Read the model definition and answer for the solid it produces. Units are mm, in the model's axes. Coordinates: 2 decimals unless noted, no trailing zeros. Loops run counter-clockwise (first coordinate to the right, second up) from the corner with the lowest first, then second, coordinate; pieces in that order, holes last.
Q1. Section D-D (x = 6.75) is taken. Give the vertices of the cut face in (y, z).
Q2. Straight lines are drawn through the part: line 1 (Z direction, x = 0.5, y = 25.5); line 2 (Y direction, x = 7.5, z = -23); line 3 (Z direction, x = 4.25, y = 12). For each, find the intervals that lie inside material, in ascending order.
Q3. Section A-A (y = 0) is taken. Give the vertices of the cut face in (x, z).
Q4. Section C-C (y = 22.5) is taken. Give the vertices of the cut face in (x, z).
Q5. The mould has two halves that part along Y. Classify faces 1 (the face through (4.056, 25.203, -22.098)), 2 (the face through (3.94, -39.05, 8.67)), 3 (the face through (0, -26.1, 9.4)), 4 (the face through (4.056, -26.846, 5.961)): pulls with the +Y half, pulls with the -Y half, needs draft (parallel to the pull), parting line crosses it, or undercut.
Q6. A flat-ended cylindrical pin translates along its axis: P1, Ø4, axis at x = 2.5, z = 12, coming from the -Y side. Find the tip coordinate at first contact, or state that the pin passes through.
from build123d import *

# Parameters (mm, degrees)
SKETCH1_R           = 40
BOSS_EXTRUDE1_DEPTH = 8
SKETCH3_R           = 4
SKETCH3_R_2         = 4.000000002
CUT_EXTRUDE1_DEPTH  = 8
SKETCH4_R           = 27.5
CUT_EXTRUDE2_DEPTH  = 8


with BuildPart() as part:
    # Sketch1 → Boss-Extrude1 (new body)
    with BuildSketch(Plane(origin=(0, 0, 0), x_dir=(0, 0, -1), z_dir=(1, 0, 0))):
        Circle(SKETCH1_R)
    extrude(amount=BOSS_EXTRUDE1_DEPTH)

    # Sketch3 → Cut-Extrude1 (cut)
    with BuildSketch(Plane(origin=(8, 0, 0), x_dir=(0, 0, -1), z_dir=(1, 0, 0))):
        with Locations((-24.95415797, 22.5)):
            Circle(SKETCH3_R)
        with Locations((25.04584203, 22.500000005)):
            Circle(SKETCH3_R_2)
        with Locations((-24.95415797, -22.5)):
            Circle(SKETCH3_R)
        with Locations((25.04584203, -22.500000005)):
            Circle(SKETCH3_R_2)
    extrude(amount=-CUT_EXTRUDE1_DEPTH, mode=Mode.SUBTRACT)

    # Sketch4 → Cut-Extrude2 (cut)
    with BuildSketch(Plane(origin=(8, 0, 0), x_dir=(0, 0, -1), z_dir=(1, 0, 0))):
        Circle(SKETCH4_R)
    extrude(amount=-CUT_EXTRUDE2_DEPTH, mode=Mode.SUBTRACT)


solid = part.part
Numbers:
1. outline: circle Ø80 at (0, 0); hole circle Ø55 at (0, 0); hole circle Ø8 at (-22.5, -25.05); hole circle Ø8 at (-22.5, 24.95); hole circle Ø8 at (22.5, -25.05); hole circle Ø8 at (22.5, 24.95)
2. line 1: z = -30.82 to -27.69, -22.4 to -10.3, 10.3 to 22.31, 27.6 to 30.82
2. line 2: y = -32.73 to -25.94, -19.06 to -15.07, 15.07 to 19.06, 25.94 to 32.73
2. line 3: z = -38.16 to -24.74, 24.74 to 38.16
3. outline: (0, -40) - (8, -40) - (8, -27.5) - (0, -27.5) - close; (0, 27.5) - (8, 27.5) - (8, 40) - (0, 40) - close
4. outline: (0, -33.07) - (8, -33.07) - (8, -29.05) - (0, -29.05) - close; (0, -21.05) - (8, -21.05) - (8, -15.81) - (0, -15.81) - close; (0, 15.81) - (8, 15.81) - (8, 20.95) - (0, 20.95) - close; (0, 28.95) - (8, 28.95) - (8, 33.07) - (0, 33.07) - close
5. face 1: undercut
5. face 2: parting line crosses it
5. face 3: needs draft
5. face 4: undercut
6. P1: stops at y = -38.73
